Build history of the part. All positions in model axes, mm. A direction names the side the tool comes from. Round coordinates to 2 decimals unless told otherwise and drop trailing zeros. Write each loop counter-clockwise with the first axis right and the second up, starting at its lowest first coordinate (ties: lowest second). Pieces come first, ordered by that corner, then holes. Notation, with made-up numbers: M 72,17.25 L 79,17.25 A16 ccw 79,22.25 Z; hole C 21.25,67.25 d10. An arc over 180 degrees is marked long. Write item = value, one per line.
from build123d import *

# Parameters (mm, degrees)
SKETCH_1_R          = 25
EXTRUDE_1_DEPTH     = 13
SKETCH_3_R          = 2
CUT_EXTRUDE_3_DEPTH = 38.669616404
SKETCH_4_R          = 19
CUT_EXTRUDE_1_DEPTH = 10
SKETCH_5_R          = 13
CUT_EXTRUDE_2_DEPTH = 38.669616404


with BuildPart() as part:
    # Эскиз1 → Вытянуть1 (new body)
    with BuildSketch(Plane(origin=(0, 0, 0), x_dir=(1, 0, 0), z_dir=(0, 1, 0))):
        with Locations(Location((0, 0, 0), (0, 0, 90))):
            Circle(SKETCH_1_R)
    extrude(amount=EXTRUDE_1_DEPTH)

    # Эскиз3 → Вытянуть3 (cut, through all)
    with BuildSketch(Plane(origin=(0, 0, 0), x_dir=(1, 0, 0), z_dir=(0, 1, 0))):
        with Locations(Location((0, 21.703286444, 0), (0, 0, 90))):
            Circle(SKETCH_3_R)
        with Locations(Location((18.795597406, 10.851643222, 0), (0, 0, 90))):
            Circle(SKETCH_3_R)
        with Locations(Location((18.795597406, -10.851643222, 0), (0, 0, 90))):
            Circle(SKETCH_3_R)
        with Locations(Location((0, -21.703286444, 0), (0, 0, 90))):
            Circle(SKETCH_3_R)
        with Locations(Location((-18.795597406, -10.851643222, 0), (0, 0, 90))):
            Circle(SKETCH_3_R)
        with Locations(Location((-18.795597406, 10.851643222, 0), (0, 0, 90))):
            Circle(SKETCH_3_R)
    extrude(amount=CUT_EXTRUDE_3_DEPTH, mode=Mode.SUBTRACT)

    # Эскиз4 → Вырез-Вытянуть1 (cut)
    with BuildSketch(Plane.XZ):
        with Locations(Location((0, 0, 0), (0, 0, 270))):
            Circle(SKETCH_4_R)
    extrude(amount=-CUT_EXTRUDE_1_DEPTH, mode=Mode.SUBTRACT)

    # Эскиз5 → Вырез-Вытянуть2 (cut, through all)
    with BuildSketch(Plane(origin=(0, 13, 0), x_dir=(1, 0, 0), z_dir=(0, 1, 0))):
        with Locations(Location((0, 0, 0), (0, 0, 270))):
            Circle(SKETCH_5_R)
    extrude(amount=-CUT_EXTRUDE_2_DEPTH, mode=Mode.SUBTRACT)


solid = part.part
1. Band-saw the part on D-D (z = -12). List the corners of the cut face in (x, y), plus the area to 3 significant figures.
Responses:
outline = M -21.93,0 L -20.43,0 L -20.43,13 L -21.93,13 Z; M -17.16,0 L -14.73,0 L -14.73,10 L -5,10 L -5,13 L -17.16,13 Z; M 5,10 L 14.73,10 L 14.73,0 L 17.16,0 L 17.16,13 L 5,13 Z; M 20.43,0 L 21.93,0 L 21.93,13 L 20.43,13 Z
area = 160 mm²
2. Probe probe 1 along X at (y, z) = (3.5, 0); probe 2 along Z at (x, y) = (-0.5, 6.5) (3 decimals); probe 3 along Z at (x, y) = (17, 8.5). List the from-to ranges inside material, lowest first.
Responses:
probe_1 = -25 to -19, 19 to 25
probe_2 = -24.995 to -23.64, -19.767 to -18.993, 18.993 to 19.767, 23.64 to 24.995
probe_3 = -18.33 to -11.73, -9.97 to -8.49, 8.49 to 9.97, 11.73 to 18.33
3. Band-saw the part on B-B (z = 0). List the corners of the cut face in (x, y), plus the area to 3 significant figures.
Responses:
outline = M -25,0 L -19,0 L -19,10 L -13,10 L -13,13 L -25,13 Z; M 13,10 L 19,10 L 19,0 L 25,0 L 25,13 L 13,13 Z
area = 192 mm²
4. Band-saw the part on A-A (x = 0). List the corners of the cut face in (y, z).
Responses:
outline = M 0,-25 L 13,-25 L 13,-23.7 L 0,-23.7 Z; M 0,-19.7 L 13,-19.7 L 13,-13 L 10,-13 L 10,-19 L 0,-19 Z; M 0,19 L 10,19 L 10,13 L 13,13 L 13,19.7 L 0,19.7 Z; M 0,23.7 L 13,23.7 L 13,25 L 0,25 Z
5. Tool access for faces 1 (the face through (-11.56, 4.93, 15.08)), 2 (the face through (20.013, 6.409, -9.265)): list every direction of +Z, -Z, +X, -X, +Y, -Y with a clear straight run to the whole face (end or side of a thin tool).
Responses:
face_1 = -Y
face_2 = +Y, -Y
6. Flat gauge pins, fed straight in: pin 1 (1 mm diameter, centred on y = 6.5, z = 17, fed in from -X); pin 2 (1.5 mm diameter, centred on y = 8.5, z = 16, fed in from +X); pin 3 (6.5 mm diameter, centred on x = 18.8, z = 10.85, fed in from -Y); pin 4 (1.5 mm diameter, centred on x = 9, y = 5.5, fed in from -Z). Where does each tip first touch, or does it go through?
Responses:
pin_1 = -18.78
pin_2 = 19.81
pin_3 = 0
pin_4 = -23.6
7. Band-saw the part on C-C (x = -6.5). List the corners of the cut face in (y, z).
Responses:
outline = M 0,-24.14 L 13,-24.14 L 13,-11.26 L 10,-11.26 L 10,-17.85 L 0,-17.85 Z; M 0,17.85 L 10,17.85 L 10,11.26 L 13,11.26 L 13,24.14 L 0,24.14 Z
